Design review of the part shown in the three views and the two pictorial views. Dimensions are in mm from the part's minimum x, y and z. Coordinates: 2 decimals unless noted, no trailing zeros. Answer as a JSON object with one key per item and string values. Group by question number.
1) For pin 1 (3.5 mm diameter, centred on y = 17.5, z = 283.5, fed in from +X); pin 2 (17 mm diameter, centred on x = 19.05, z = 222.25, fed in from -Y), all flat-tipped, find the tip position at first contact; note any pin that passes through.
2) Wall thickness on L1, parallel to Z at x = 19.05, y = 16.9; L2, parallel to Z at x = 19.05, y = 1.2; L3, parallel to X at y = 17.2, z = 222.25: over which ranges is each line inside the solid? List them lowest first.
3) Draft analysis for pull direction Y (two halves, no side actions). For the marked faces 1 and 2, state which applies: +Y half, -Y half, draft (parallel to the pull), parting line (faces both ways), or undercut.
4) Add section D-D, the plane x = 19.05. Count the separate pieces of the cut face and the enclosed holes in it.
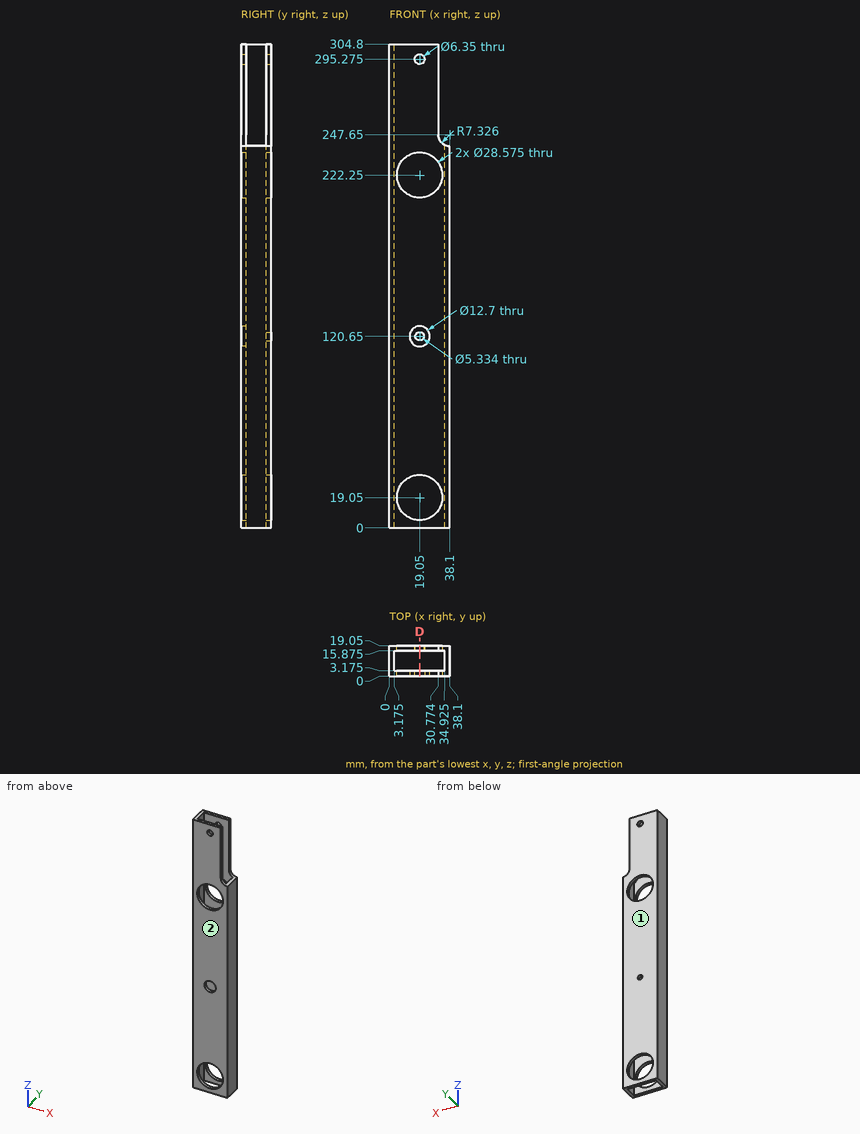
Output values:
{
 "1": {"pin 1": "stops at x = 30.77", "pin 2": "passes through"},
 "2": {"L1": "z = 0 to 4.76, 33.34 to 117.98, 123.32 to 207.96, 236.54 to 292.1, 298.45 to 304.8", "L2": "z = 0 to 4.76, 33.34 to 114.3, 127 to 207.96, 236.54 to 292.1, 298.45 to 304.8", "L3": "x = 0 to 4.76, 33.34 to 38.1"},
 "3": {"face 1": "+Y half", "face 2": "-Y half"},
 "4": {"separate pieces": "10", "enclosed holes": "0"}
}
